Could you check a few things on this model? Use its own coordinates, in mm. A direction names the side the tool comes from. Round coordinates to 2 decimals unless told otherwise and drop trailing zeros. Write each loop counter-clockwise with the first axis right and the second up, starting at its lowest first coordinate (ties: lowest second). Pieces come first, ordered by that corner, then holes. Notation, with made-up numbers: M -12.5,79.5 L -6.5,79.5 A14 cw -6.5,87.5 Z; hole C 19.5,45.25 d1. An arc over 180 degrees is marked long. One line per item, written item: value. Start each with the question number.
(1) If I drill on L1, parallel to X at y = 2.25, z = 7.25; L2, parallel to Z at x = 2.5, y = 0.25; L3, parallel to X at y = 1, z = 0, over which ranges is the centre line in solid material (lowest first)?
(2) I want a section at A-A on z = 3.5. Please give me the cut outline in (x, y), and give its area (3 significant figures).
(3) Which directions (+Z, -Z, +X, -X, +Y, -Y) give clear straight access to the entire face, cutting with the end or side of a thin tool? Please do faces 1 (the face through (0, 0, 8)), 2 (the face through (1.3, -1.3, 6)).
(4) I'm going to push flat-ended pins straight in: pin 1 Ø1 at (x, z) = (-0.5, -0.5) entering from -Y; pin 2 Ø2 at (x, y) = (2.5, -1) entering from +Z. Where does each tip first touch, or does it pass through?
Autodesk Inventor part; units mm, degrees
ref_plane "YZ Plane" through (0, 0, 0) normal (1, 0, 0) x (0, 1, 0)
ref_plane "XZ Plane" through (0, 0, 0) normal (0, 1, 0) x (-1, 0, 0)
ref_plane "XY Plane" through (0, 0, 0) normal (0, 0, 1) x (1, 0, 0)
sketch "スケッチ1" plane through (0, 0, 0) normal (0, 0, 1) x (1, 0, 0)
  circle A0 centre (0, 0) radius 1.5
  dimension "d0" = 3
extrude "押し出し1" add sketch "スケッチ1" along normal blind 6
sketch "スケッチ2" plane through (0, 0, 6) normal (0, 0, 1) x (1, 0, 0)
  circle A0 centre (0, 0) radius 1.5
  circle A1 centre (0, 0) radius 3
  dimension "d3" = 6
extrude "押し出し2" add sketch "スケッチ2" along normal blind 2 contours A0 | A1
fillet "フィレット1" radius 2 1 edges at (-3, 0, 8)
thread "ねじ1"
sketch "スケッチ3" plane through (0, 0, 0) normal (0, 0, -1) x (-1, 0, 0)
  circle A0 centre (0, 0) radius 1.5
extrude "押し出し3" add sketch "スケッチ3" along normal blind 2
sketch "スケッチ4" plane through (0, 0, -2) normal (0, 0, -1) x (-1, 0, 0)
  circle A0 centre (0, 0) radius 1.5
extrude "押し出し4" add sketch "スケッチ4" along normal blind 2
properties part number "SB　10mmなべネジ" material "Steel, Mild"
Found:
1. L1: x = -1.22 to 1.22
1. L2: z = 6 to 7.31
1. L3: x = -1.12 to 1.12
2. outline: C 0,0 d3
2. area: 7.07 mm²
3. face 1: +Z, +X, -X, +Y, -Y
3. face 2: -Z
4. pin 1: stops at y = -1.5
4. pin 2: stops at z = 7.88
